Could you check a few things on this model? Use its own coordinates, in mm. A direction names the side the tool comes from. Coordinates: 2 decimals unless noted, no trailing zeros. Loops run counter-clockwise (first coordinate to the right, second up) from the corner with the lowest first, then second, coordinate; pieces in that order, holes last.
from build123d import *

# Parameters (mm, degrees)
BOSS_EXTRUDE1_DEPTH = 2.5


with BuildPart() as part:
    # Sketch1 → Boss-Extrude1 (new, symmetric)
    with BuildSketch(Plane(origin=(0, 0, 0), x_dir=(-1, 0, 0), z_dir=(0, 1, 0))):
        with BuildLine():
            ThreePointArc((0, 15.875), (11.225320151, 11.225320151), (15.875, 0))
            Line((15.875, 0), (163.044989153, 0))
            Line((163.044989153, 0), (163.044989153, 10.875))
            Line((163.044989153, 10.875), (157.04, 10.875))
            Line((157.04, 10.875), (157.04, 15.875))
            Line((157.04, 15.875), (147.04, 15.875))
            Line((147.04, 15.875), (147.04, 10.875))
            Line((147.04, 10.875), (141.04, 10.875))
            Line((141.04, 10.875), (141.04, 5.875))
            Line((141.04, 5.875), (136.04, 5.875))
            Line((136.04, 5.875), (136.04, 10.875))
            Line((136.04, 10.875), (100, 10.875))
            Line((100, 10.875), (100, 15.875))
            Line((100, 15.875), (0, 15.875))
        make_face()
    extrude(amount=BOSS_EXTRUDE1_DEPTH, both=True)


solid = part.part
(1) We'd pull the mould along X, two halves only. Please class faces 1 (the face through (-163.045, 0, 5)), 2 (the face through (-136.04, 0, 8)), 3 (the face through (-160, 0, 10.875)): +X half, -X half, draft (parallel to the pull), parting line (faces both ways), or undercut.
Answers:
face 1: -X half
face 2: undercut
face 3: draft
(2) I need wall thicknesses on probe 1 along Z at (x, y) = (-110, -0.55) (3 decimals); probe 2 along X at (y, z) = (1.9, 9.5); probe 3 along X at (y, z) = (-1.3, 11). Which ranges of each line are inside material? Lowest first, please.
Answers:
probe 1: z = 0 to 10.875
probe 2: x = -163.04 to -141.04, -136.04 to -12.72
probe 3: x = -157.04 to -147.04, -100 to -11.45
(3) Imagine slicing it at D-D, the plane z = 4.25. Write out the boundary of the cut face in (x, y), and give its area (3 significant figures).
Answers:
outline: (-163.04, -2.5) - (-15.3, -2.5) - (-15.3, 2.5) - (-163.04, 2.5) - close
area: 739 mm2
(4) Imagine slicing it at A-A, the plane z = 13.75. Write out the boundary of the cut face in (x, y), and give its area (3 significant figures).
Answers:
outline: (-157.04, -2.5) - (-147.04, -2.5) - (-147.04, 2.5) - (-157.04, 2.5) - close; (-100, -2.5) - (-7.93, -2.5) - (-7.93, 2.5) - (-100, 2.5) - close
area: 510 mm2
(5) Imagine slicing it at C-C, the plane x = -134. Write out the boundary of the cut face in (y, z) (3 decimals).
Answers:
outline: (-2.5, 0) - (2.5, 0) - (2.5, 10.875) - (-2.5, 10.875) - close
(6) Which directions (+Z, -Z, +X, -X, +Y, -Y) give clear straight access to the entire face, cutting with the end or side of a thin tool? Please do faces 4 (the face through (-157.04, 0, 13)), 5 (the face through (-11.1, 0.04, 11.35)), 6 (the face through (-139, 0, 5.875)).
Answers:
face 4: +Z, -X, +Y, -Y
face 5: -Z, +X, +Y, -Y
face 6: +Z, +Y, -Y
(7) For pin 1 (1.5 mm diameter, centred on y = 0.5, z = 8.5, fed in from +X); pin 2 (2 mm diameter, centred on y = -1, z = 7, fed in from +X); pin 3 (2.5 mm diameter, centred on x = -137.5, y = -0.5, fed in from +Z) (3 decimals), each with a flat end and sliding along its axis, tell me the tip position at first contact or that it passes through.
Answers:
pin 1: stops at x = -12.9
pin 2: stops at x = -13.71
pin 3: stops at z = 5.875
(8) Imagine slicing it at B-B, the plane y = 0.4. Write out the boundary of the cut face in (x, z) (3 decimals).
Answers:
outline: (-163.045, 0) - (-15.875, 0) arc R15.875 cw to (0, 15.875) - (-100, 15.875) - (-100, 10.875) - (-136.04, 10.875) - (-136.04, 5.875) - (-141.04, 5.875) - (-141.04, 10.875) - (-147.04, 10.875) - (-147.04, 15.875) - (-157.04, 15.875) - (-157.04, 10.875) - (-163.045, 10.875) - close
